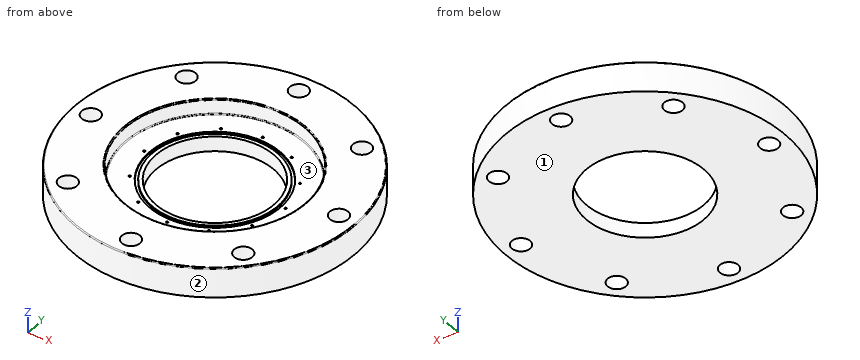
from build123d import *

# Parameters (mm, degrees)
SKETCH1_R          = 171.45
EXTRUDE1_DEPTH     = 36.5125
SKETCH2_R          = 11.1125
EXTRUDE2_DEPTH     = 246.20066814
CIRPATTERN1_COUNT  = 8
FILLET1_R          = 1.154545455
SKETCH4_R          = 72
CUT_EXTRUDE1_DEPTH = 120
CIRPATTERN2_COUNT  = 12
SKETCH5_R          = 80
SKETCH5_R_2        = 76.5
CUT_EXTRUDE2_DEPTH = 2


with BuildPart() as part:
    # Sketch1 → Extrude1 (new body)
    with BuildSketch(Plane.XY):
        Circle(SKETCH1_R)
    extrude(amount=EXTRUDE1_DEPTH)

    # Sketch2 → Extrude2 (cut, through all)
    with BuildSketch(Plane.XY.offset(36.5125)):
        with Locations((0, 149.225)):
            Circle(SKETCH2_R)
    extrude2 = extrude(amount=-EXTRUDE2_DEPTH, mode=Mode.SUBTRACT)

    # CirPattern1: Extrude2 ×8 about axis
    cirpattern1_axis = Axis((0, 0, 0), (0, 0, 1))
    for i in range(1, CIRPATTERN1_COUNT):
        add(extrude2.rotate(cirpattern1_axis, i * 360 / CIRPATTERN1_COUNT), mode=Mode.SUBTRACT)

    # Sketch3 → Cut-Revolve1 (revolve, cut)
    with BuildSketch(Plane(origin=(0, 0, 0), x_dir=(0, 0, -1), z_dir=(1, 0, 0))):
        Polygon((-36.5125, 109.9185), (-18.25625, 109.347), (-18.25625, 0), (-36.5125, 0), align=None)
    revolve(axis=Axis((0, 0, 18.25625), (0, 0, 1)), mode=Mode.SUBTRACT)

    # Fillet1
    fillet1_edges = [part.edges().sort_by_distance(p)[0] for p in [
        (0, -109.347, 18.25625),
        (0, -109.9185, 36.5125),
        (-171.45, 0, 36.5125),
    ]]
    fillet(fillet1_edges, radius=FILLET1_R)

    # Sketch4 → Cut-Extrude1 (cut)
    with BuildSketch(Plane(origin=(0, 0, 0), x_dir=(-1, 0, 0), z_dir=(0, 0, -1))):
        Circle(SKETCH4_R)
    extrude(amount=-CUT_EXTRUDE1_DEPTH, mode=Mode.SUBTRACT)

    # Sketch8 → M3x0.5 Tapped Hole1 (revolve, cut)
    with BuildSketch(Plane(origin=(0, 85, 18.25625), x_dir=(0, -1, 0), z_dir=(1, 0, 0))):
        Polygon((0, 0), (0, 12.751075774), (1.25, 12), (1.25, 0), align=None)
    m3x0_5_tapped_hole1 = revolve(axis=Axis((0, 85, 24.60625), (0, 0, -1)), mode=Mode.SUBTRACT)

    # CirPattern2: M3x0.5 Tapped Hole1 ×12 about axis
    cirpattern2_axis = Axis((0, 0, 0), (0, 0, 1))
    for i in range(1, CIRPATTERN2_COUNT):
        add(m3x0_5_tapped_hole1.rotate(cirpattern2_axis, i * 360 / CIRPATTERN2_COUNT), mode=Mode.SUBTRACT)

    # Sketch5 → Cut-Extrude2 (cut)
    with BuildSketch(Plane(origin=(0, 0, 18.25625), x_dir=(-1, 0, 0), z_dir=(0, 0, -1))):
        Circle(SKETCH5_R)
        Circle(SKETCH5_R_2, mode=Mode.SUBTRACT)
    extrude(amount=CUT_EXTRUDE2_DEPTH, mode=Mode.SUBTRACT)


solid = part.part
Could you check a few things on this model? Use its own coordinates, in mm. Face numbers are marked on the shaded views. Round coordinates to 2 decimals unless told otherwise and drop trailing zeros.
Q1. Thinking about a two-plate mould opening in Y: for the marked faces 1, 2 and 3, which applies, released by +Y, released by -Y, zero draft, split by the parting line, or undercut?
Geometry says:
face 1: zero draft
face 2: split by the parting line
face 3: undercut
Q2. Imagine slicing it at A-A, the plane z = 31. State how many separate pieces and enclosed holes the cut face has, then the cut area to 3 significant figures.
Geometry says:
separate pieces: 1
enclosed holes: 9
area: 51,400 mm2
Q3. Please list where these lines run through material, in increasing order: probe 1 along Y at (x, z) = (0, 9.5); probe 2 along Y at (x, z) = (0, 22); probe 3 along X at (y, z) = (-99, 17).
Geometry says:
probe 1: y = -171.45 to -160.34, -138.11 to -86.25, -83.75 to -72, 72 to 83.75, 86.25 to 138.11, 160.34 to 171.45
probe 2: y = -171.45 to -160.34, -138.11 to -109.46, 109.46 to 138.11, 160.34 to 171.45
probe 3: x = -139.98 to -114.52, -96.52 to 96.52, 114.52 to 139.98
Q4. I'm going to push flat-ended pins straight in: P1, Ø2, axis at x = -131, z = 16.5, coming from the +Y side; P2, Ø20, axis at x = -105.52, y = 105.52, coming from the +Z side; P3, Ø1, axis at x = -94.5, z = 9, coming from the +Y side; P4, Ø2, axis at x = 73.61, y = 42.5, coming from the +Z side. Where does each tip first touch, or does it pass through?
Geometry says:
P1: stops at y = 111.78
P2: passes through
P3: stops at y = 143.38
P4: stops at z = 6.11
